CAD build for the part. Positions are in the model's coordinates, mm. A direction names the side the tool comes from. Give positions to 0.01 mm unless a question says otherwise; leave off trailing zeros. Loops run counter-clockwise (first coordinate to the right, second up) from the corner with the lowest first, then second, coordinate; pieces in that order, holes last. Notation, with made-up numbers: M 69.25,22.5 L 77.25,22.5 A29 cw 77.25,61.5 Z; hole C -8,-37 d3. An arc over 180 degrees is marked long. One line per question, with ' | ' between items.
```python
from build123d import *

# Parameters (mm, degrees)
SKETCH1_W           = 20
SKETCH1_H           = 60
BOSS_EXTRUDE1_DEPTH = 5
SKETCH2_R           = 2.5
SKETCH2_R_2         = 1.25
BOSS_EXTRUDE2_DEPTH = 20
SKETCH3_R           = 1.25
CUT_EXTRUDE1_DEPTH  = 29
SKETCH4_R           = 2.5
SKETCH4_R_2         = 1.25
BOSS_EXTRUDE3_DEPTH = 20
SKETCH5_R           = 1.25
CUT_EXTRUDE2_DEPTH  = 29
SKETCH6_R           = 1.25
BOSS_EXTRUDE4_DEPTH = 30
SKETCH7_W           = 20.6
SKETCH7_H           = 7
CUT_EXTRUDE3_DEPTH  = 30
SKETCH8_W           = 60.511546569
SKETCH8_H           = 78.563917263
CUT_EXTRUDE4_DEPTH  = 41
SKETCH10_W          = 60
SKETCH10_H          = 5
BOSS_EXTRUDE5_DEPTH = 5
SKETCH11_R          = 1.012314422
CUT_EXTRUDE5_DEPTH  = 41


with BuildPart() as part:
    # Sketch1 → Boss-Extrude1 (new body)
    with BuildSketch(Plane.XY):
        with Locations((10, 30)):
            Rectangle(SKETCH1_W, SKETCH1_H)
    extrude(amount=BOSS_EXTRUDE1_DEPTH)

    # Sketch2 → Boss-Extrude2 (add)
    with BuildSketch(Plane(origin=(20, 0, 0), x_dir=(0, 0, -1), z_dir=(1, 0, 0))):
        with Locations((-2.5, 60)):
            Circle(SKETCH2_R)
        with Locations((-2.5, 60)):
            Circle(SKETCH2_R_2, mode=Mode.SUBTRACT)
    extrude(amount=-BOSS_EXTRUDE2_DEPTH)

    # Sketch3 → Cut-Extrude1 (cut)
    with BuildSketch(Plane.ZY):
        with Locations(Location((2.5, 60, 0), (0, 0, 180))):
            Circle(SKETCH3_R)
    extrude(amount=-CUT_EXTRUDE1_DEPTH, mode=Mode.SUBTRACT)

    # Sketch4 → Boss-Extrude3 (add)
    with BuildSketch(Plane.ZY):
        with Locations((2.5, 0)):
            Circle(SKETCH4_R)
        with Locations((2.5, 0)):
            Circle(SKETCH4_R_2, mode=Mode.SUBTRACT)
    extrude(amount=-BOSS_EXTRUDE3_DEPTH)

    # Sketch5 → Cut-Extrude2 (cut)
    with BuildSketch(Plane(origin=(20, 0, 0), x_dir=(0, 0, -1), z_dir=(1, 0, 0))):
        with Locations(Location((-2.5, 0, 0), (0, 0, 180))):
            Circle(SKETCH5_R)
    extrude(amount=-CUT_EXTRUDE2_DEPTH, mode=Mode.SUBTRACT)

    # Sketch6 → Boss-Extrude4 (add)
    with BuildSketch(Plane.ZY):
        with BuildLine():
            Line((5, 60), (5, 70))
            Line((5, 70), (0, 70))
            Line((0, 70), (0, 60))
            ThreePointArc((0, 60), (2.5, 57.5), (5, 60))
        make_face()
        with Locations(Location((2.5, 60, 0), (0, 0, 180))):
            Circle(SKETCH6_R, mode=Mode.SUBTRACT)
    extrude(amount=BOSS_EXTRUDE4_DEPTH)

    # Sketch7 → Cut-Extrude3 (cut)
    with BuildSketch(Plane(origin=(0, 0, 0), x_dir=(-1, 0, 0), z_dir=(0, 0, -1))):
        with Locations((15, 60)):
            Rectangle(SKETCH7_W, SKETCH7_H)
    extrude(amount=-CUT_EXTRUDE3_DEPTH, mode=Mode.SUBTRACT)

    # Sketch8 → Cut-Extrude4 (cut)
    with BuildSketch(Plane.ZY):
        with Locations((2.066743104, 31.078249137)):
            Rectangle(SKETCH8_W, SKETCH8_H)
    extrude(amount=-CUT_EXTRUDE4_DEPTH, mode=Mode.SUBTRACT)

    # Sketch10 → Boss-Extrude5 (add)
    with BuildSketch(Plane(origin=(0, 0, 0), x_dir=(-1, 0, 0), z_dir=(0, 0, -1))):
        with Locations((15, 70.5)):
            Rectangle(SKETCH10_W, SKETCH10_H)
    extrude(amount=-BOSS_EXTRUDE5_DEPTH)

    # Sketch11 → Cut-Extrude5 (cut)
    with BuildSketch(Plane(origin=(0, 0, 0), x_dir=(-1, 0, 0), z_dir=(0, 0, -1))):
        with Locations(Location((-12.5, 70.5, 0), (0, 0, 90))):
            Circle(SKETCH11_R)
        with Locations(Location((42.5, 70.5, 0), (0, 0, 90))):
            Circle(SKETCH11_R)
    extrude(amount=-CUT_EXTRUDE5_DEPTH, mode=Mode.SUBTRACT)


solid = part.part
```
Item 1: 3-axis set-ups, long thin cutter, end or side, ignore diameter. For faces 1 (the flat face through (-30, 63, 2)), 2 (the flat face through (8, 68, 2)), 3 (the flat face through (-4.7, 62, 2)): which of +Z, -Z, +X, -X, +Y, -Y reach the whole face in a straight line?
Conclusion:
face 1: +Z, -Z, -X, -Y | face 2: +Z, -Z, +X, -Y | face 3: +Z, -Z, -Y
Item 2: Drill centre lines: line 1 along X through (y, z) = (70.5, 2.45); line 2 along Z through (x, y) = (-27.8, 60); line 3 along Y through (x, z) = (-26.3, 2.5). Where is each one in solid material? Low to high. Write a range as [from, to].
Conclusion:
line 1: [-45, -43.51], [-41.49, 11.49], [13.51, 15] | line 2: [0, 1.25], [3.75, 5] | line 3: [57.5, 58.75], [61.25, 73]
Item 3: Saw through at C-C on y = 70.5. Give the cut face in (x, z).
Conclusion:
outline: M -45,0 L -43.51,0 L -43.51,5 L -45,5 Z; M -41.49,0 L 11.49,0 L 11.49,5 L -41.49,5 Z; M 13.51,0 L 15,0 L 15,5 L 13.51,5 Z
Item 4: Saw through at D-D on x = 9.5. Give the cut face in (y, z), and give its area (3 significant figures).
Conclusion:
outline: M 68,0 L 73,0 L 73,5 L 68,5 Z | area: 25.0 mm²
Item 5: Drop flat-ended pins along their axis: P1, Ø2, axis at y = 65, z = 1, coming from the +X side; P2, Ø2, axis at x = -38.5, z = 3.5, coming from the -Y side; P3, Ø2.5, axis at x = -13.5, z = 3.5, coming from the -Y side. Give the stop position or say it passes through.
Conclusion:
P1: x = 0 | P2: y = 68 | P3: y = 63.5
Item 6: Saw through at B-B on x = -42.5. Give the cut face in (y, z).
Conclusion:
outline: M 68,0 L 69.49,0 L 69.49,5 L 68,5 Z; M 71.51,0 L 73,0 L 73,5 L 71.51,5 Z
Item 7: Saw through at A-A on z = 2.5. Give the cut face in (x, y), and give its area (3 significant figures).
Conclusion:
outline: M -45,68 L -30,68 L -30,61.25 L -25.3,61.25 L -25.3,63.5 L -4.7,63.5 L -4.7,61.25 L 0,61.25 L 0,68 L 15,68 L 15,73 L -45,73 Z; M -30,57.5 L -25.3,57.5 L -25.3,58.75 L -30,58.75 Z; M -4.7,57.5 L 0,57.5 L 0,58.75 L -4.7,58.75 Z; hole C -42.5,70.5 d2.02; hole C 12.5,70.5 d2.02 | area: 461 mm²
Item 8: Mould opens along Y. For faces 4 (the flat face through (-37, 68, 2)), 5 (the cylindrical face through (-27.62, 58.76, 2.66)), 6 (the flat face through (-15, 68, 0)) say: pulls with the +Y half, pulls with the -Y half, needs draft (parallel to the pull), parting line crosses it, or undercut.
Conclusion:
face 4: pulls with the -Y half | face 5: undercut | face 6: needs draft
